```python
from build123d import *

# Parameters (mm, degrees)
F0_W      = 145.415
F0_H      = 15.875
F1_DEPTH  = 25.4
F3_DEPTH  = 25.4
F2_R      = 3.9042600658
F4_DEPTH  = 3.302
F5_W      = 10.0848590955
F5_H      = 7.6029407792
F6_DEPTH  = 25.4
F7_W      = 3.4926307648
F7_H      = 25.4
F9_R      = 4.1220063289
F10_DEPTH = 25.4


with BuildPart() as f1:
    # F0 (on Top) → F1 (new body)
    with BuildSketch(Plane.XY):
        Rectangle(F0_W, F0_H)
    extrude(amount=F1_DEPTH)

    # F2 (on face) → F3 (join)
    with BuildSketch(Plane.XY.offset(25.4)):
        with BuildLine():
            ThreePointArc((-38.4175, 7.9375), (-37.4473063314, -2.8221126628), (-28.2575, 2.8575))
            ThreePointArc((-28.2575, 2.8575), (-28.9278873372, 5.6973063314), (-30.7975, 7.9375))
            Line((-30.7975, 7.9375), (-38.4175, 7.9375))
        make_face()
    extrude(amount=F3_DEPTH)

    # F2 (on face) → F4 (cut)
    with BuildSketch(Plane.XY.offset(25.4)):
        with Locations((-60.1726733148, 0)):
            Circle(F2_R)
    extrude(amount=-F4_DEPTH, mode=Mode.SUBTRACT)

    # F5 (on face) → F6 (cut, through all)
    with BuildSketch(Plane.XY.offset(25.4)):
        with Locations((-8.0950618722, -0.9069514927)):
            Rectangle(F5_W, F5_H)
    extrude(amount=-F6_DEPTH, mode=Mode.SUBTRACT)

    # F7 (on face) → F8 (revolve)
    with BuildSketch(Plane.YZ.offset(72.7075)):
        with Locations((6.1911846176, 12.7)):
            Rectangle(F7_W, F7_H)
    revolve(axis=Axis((72.7075, 7.9375, 12.7), (0, 0, -1)))

    # F9 (on face) → F10 (join, through all)
    with BuildSketch(Plane.XY.offset(25.4)):
        with Locations((72.7075, -7.9375)):
            Circle(F9_R)
    extrude(amount=-F10_DEPTH)


solid = f1.part
```
For this review, take the finished solid that the model builds, in its own axes (mm). A direction names the side the tool comes from. Round coordinates to 2 decimals unless told otherwise and drop trailing zeros. Write each loop counter-clockwise with the first axis right and the second up, starting at its lowest first coordinate (ties: lowest second). Pieces come first, ordered by that corner, then holes. Notation, with made-up numbers: M -25,26 L -10,26 A13 cw -10,42 Z; hole C 39,75 d11. An arc over 180 degrees is marked long. One line per item, written item: value. Start each with the question number.
(1) We need section D-D (y = -10.25). Give the boundary of the cut face in (x, z).
(2) Wall thickness on line 1 (Y direction, x = -7, z = 3); line 2 (Z direction, x = -24, y = 4); line 3 (Y direction, x = -24, z = 12): over which ranges is each line inside the solid? List them lowest first.
(3) Machinability: for faces 4 (the flat face through (-3, 7.938, 14)), 5 (the flat face through (-60, 0, 22.098)), 6 (the flat face through (-3, -7.938, 13)), which of the approach directions +Z, -Z, +X, -X, +Y, -Y give a long, thin tool a straight path to every point of the face, cutting with its end or side? Answer none if there is none.
(4) The part is to be moulded in two halves that separate along X. For faces 1 (the cylindrical face through (75.09, 10.49, 12.88)), 2 (the flat face through (72.708, 0, 13)), 3 (the flat face through (-3.053, -1, 13)), say which applies: released by +X, released by -X, zero draft, split by the parting line, or undercut.
(5) Insertion check: pin 1 (8.5 mm diameter, centred on y = -2, z = 15, fed in from +X); pin 2 (12.5 mm diameter, centred on x = 16.5, z = 9, fed in from -Y); pin 3 (7 mm diameter, centred on x = 34.5, y = 1.5, fed in from +Z); pin 4 (6 mm diameter, centred on x = 48, y = 4.5, fed in from -Z). Each pin has a flat end and moves straight along its axis. Give the tip position at first contact, or say it passes through.
(6) We need section C-C (x = -58). Give the boundary of the cut face in (y, z).
(7) We need section B-B (y = 0). Give the boundary of the cut face in (x, z), and give its area (3 significant figures).
(8) We need section A-A (z = 17.5). Give the boundary of the cut face in (x, y).
Result:
1. outline: M 69.3,0 L 76.12,0 L 76.12,25.4 L 69.3,25.4 Z
2. line 1: -7.94 to -4.71, 2.89 to 7.94
2. line 2: 0 to 25.4
2. line 3: -7.94 to 7.94
3. face 4: +Z, -Z, -X, +Y
3. face 5: +Z
3. face 6: +Z, -Z, -X, -Y
4. face 1: split by the parting line
4. face 2: released by +X
4. face 3: undercut
5. pin 1: x = 76.47
5. pin 2: y = -7.94
5. pin 3: z = 25.4
5. pin 4: z = 0
6. outline: M -7.94,0 L 7.94,0 L 7.94,25.4 L 3.24,25.4 L 3.24,22.1 L -3.24,22.1 L -3.24,25.4 L -7.94,25.4 Z
7. outline: M -72.71,0 L -13.14,0 L -13.14,25.4 L -28.94,25.4 L -28.94,50.8 L -40.28,50.8 L -40.28,25.4 L -56.27,25.4 L -56.27,22.1 L -64.08,22.1 L -64.08,25.4 L -72.71,25.4 Z; M -3.05,0 L 72.71,0 L 72.71,25.4 L -3.05,25.4 Z
7. area: 3,700 mm²
8. outline: M -72.71,-7.94 L 68.59,-7.94 A4.12 ccw long 72.71,-3.82 L 72.71,4.44 A3.49 ccw long 69.21,7.94 L -72.71,7.94 Z; hole M -13.14,-4.71 L -3.05,-4.71 L -3.05,2.89 L -13.14,2.89 Z
